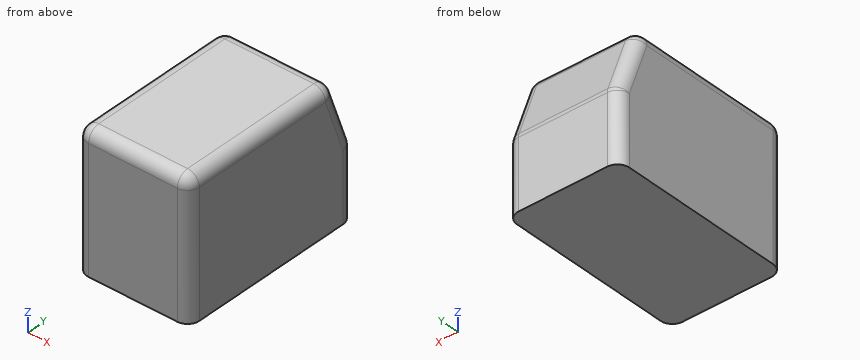
```python
from build123d import *

# Parameters (mm, degrees)
F1_DEPTH = 241.3
F2_R     = 25.4


with BuildPart() as f1:
    # F0 (on Right) → F1 (new body)
    with BuildSketch(Plane.YZ):
        Polygon((203.2, 6.35), (152.4, 146.05), (-203.2, 146.05), (-203.2, -146.05), (203.2, -146.05), align=None)
    extrude(amount=F1_DEPTH)

    # F2
    f2_edges = [f1.edges().sort_by_distance(p)[0] for p in [
        (0, -25.4, 146.05),
        (120.65, -203.2, 146.05),
        (241.3, -25.4, 146.05),
        (120.65, 152.4, 146.05),
        (0, 177.8, 76.2),
        (0, 203.2, -69.85),
        (0, -203.2, 0),
        (241.3, -203.2, 0),
        (241.3, 177.8, 76.2),
        (241.3, 203.2, -69.85),
        (120.65, 203.2, 6.35),
    ]]
    fillet(f2_edges, radius=F2_R)


solid = f1.part
```
Verification items for the finished model (mm, model axes). Coordinates: 2 decimals unless noted, no trailing zeros. Loops run counter-clockwise (first coordinate to the right, second up) from the corner with the lowest first, then second, coordinate; pieces in that order, holes last. Notation, with made-up numbers: (-33.5, 74) -> (9.5, 74) arc R19 ccw to (9.5, 89) -> close; hole circle Ø6 at (66, 5). An arc over 180 degrees is marked (long way). Put each result on its own line as item: value.
1. Gauge pin test, flat ends, axial feed: P1, Ø2, axis at x = 212, z = 80, coming from the +Y side; P2, Ø6, axis at x = 159.5, z = 47.5, coming from the +Y side; P3, Ø8, axis at x = 189, z = 96, coming from the +Y side. Record the tip position at first contact, or that the pin passes through.
Result set:
P1: stops at y = 176.78
P2: stops at y = 189.33
P3: stops at y = 172.05
2. Section check A-A, the plane x = 177. Record the boundary of the cut face in (y, z), then the cut area to 3 significant figures.
Result set:
outline: (-203.2, -146.05) -> (203.2, -146.05) -> (203.2, 1.88) arc R25.4 ccw to (201.67, 10.56) -> (158.48, 129.33) arc R25.4 ccw to (134.61, 146.05) -> (-177.8, 146.05) arc R25.4 ccw to (-203.2, 120.65) -> close
area: 115,000 mm^2
3. Thickness scan on line 1 (Y direction, x = 68, z = 43); line 2 (Y direction, x = 126, z = 11); line 3 (Z direction, x = 16.5, y = -125.5). Record the ranges inside material, lowest first.
Result set:
line 1: y = -203.2 to 189.87
line 2: y = -203.2 to 201.51
line 3: z = -146.05 to 144.44
